CAD build for the part. Positions are in the model's coordinates, mm. Coordinates: 2 decimals unless noted, no trailing zeros. Loops run counter-clockwise (first coordinate to the right, second up) from the corner with the lowest first, then second, coordinate; pieces in that order, holes last.
1) Saw through at B-B, the plane y = 50. Write the cut outline in (x, z).
2) Saw through at A-A, the plane z = 0.8. Give the number of separate pieces and of enclosed holes in the cut face, and give its area (3 significant figures).
3) Pin check, flat tip, straight feed: pin 1 Ø8 at (x, y) = (63.5, 78) entering from -Z. Stop position of the tip, or through.
4) Wall check: line 1 along Y through (x, z) = (-100, 2.5); line 2 along X through (y, z) = (-162.5, 1.65); line 3 along Y through (x, z) = (-85, 1.7). Give the ranges that are in metal, low to high.
```python
from build123d import *

# Parameters (mm, degrees)
SKETCH1_W           = 250
SKETCH1_H           = 365
BOSS_EXTRUDE1_DEPTH = 3
SKETCH3_R           = 2
CUT_EXTRUDE2_DEPTH  = 3
SKETCH4_W           = 32
SKETCH4_H           = 38
CUT_EXTRUDE3_DEPTH  = 10


with BuildPart() as part:
    # Sketch1 → Boss-Extrude1 (new body)
    with BuildSketch(Plane.XY):
        Rectangle(SKETCH1_W, SKETCH1_H)
    extrude(amount=BOSS_EXTRUDE1_DEPTH)

    # Sketch3 → Cut-Extrude2 (cut)
    with BuildSketch(Plane.XY.offset(3)):
        with Locations((-85, 167.5)):
            Circle(SKETCH3_R)
        with Locations((-85, 47.5)):
            Circle(SKETCH3_R)
        with Locations((-85, -72.5)):
            Circle(SKETCH3_R)
        with Locations((-85, -192.5)):
            Circle(SKETCH3_R)
        with Locations((85, -192.5)):
            Circle(SKETCH3_R)
        with Locations(Location((85, -72.5, 0), (0, 0, 180))):
            Circle(SKETCH3_R)
        with Locations(Location((85, 47.5, 0), (0, 0, 180))):
            Circle(SKETCH3_R)
        with Locations(Location((85, 167.5, 0), (0, 0, 180))):
            Circle(SKETCH3_R)
    extrude(amount=-CUT_EXTRUDE2_DEPTH, mode=Mode.SUBTRACT)

    # Sketch4 → Cut-Extrude3 (cut)
    with BuildSketch(Plane(origin=(0, 0, 0), x_dir=(-1, 0, 0), z_dir=(0, 0, -1))):
        with Locations((-85, -153.5)):
            Rectangle(SKETCH4_W, SKETCH4_H)
        with Locations((85, -153.5)):
            Rectangle(SKETCH4_W, SKETCH4_H)
        with Locations((-85, 46.5)):
            Rectangle(SKETCH4_W, SKETCH4_H)
        with Locations((85, 46.5)):
            Rectangle(SKETCH4_W, SKETCH4_H)
    extrude(amount=-CUT_EXTRUDE3_DEPTH, mode=Mode.SUBTRACT)


solid = part.part
```
Data:
1. outline: (-125, 0) - (-101, 0) - (-101, 3) - (-125, 3) - close; (-69, 0) - (69, 0) - (69, 3) - (-69, 3) - close; (101, 0) - (125, 0) - (125, 3) - (101, 3) - close
2. separate pieces: 1
2. enclosed holes: 8
2. area: 86,300 mm2
3. pin 1: stops at z = 0
4. line 1: y = -182.5 to -172.5, -134.5 to 27.5, 65.5 to 182.5
4. line 2: x = -125 to -101, -69 to 69, 101 to 125
4. line 3: y = -182.5 to -172.5, -134.5 to -74.5, -70.5 to 27.5, 65.5 to 165.5, 169.5 to 182.5
